Build history of the part. All positions in model axes, mm. A direction names the side the tool comes from. Round coordinates to 2 decimals unless told otherwise and drop trailing zeros. Write each loop counter-clockwise with the first axis right and the second up, starting at its lowest first coordinate (ties: lowest second). Pieces come first, ordered by that corner, then holes.
Item 1: 3-axis set-ups, long thin cutter, end or side, ignore diameter. For faces 4 (the flat face through (13, 17, -12)), 5 (the flat face through (0, 10, -10)), 6 (the conical face through (6.45, -4.125, -7.012)), 7 (the cylindrical face through (-11.77, 35.63, 9.85)), 8 (the flat face through (0, -6, -3)): which of +Z, -Z, +X, -X, +Y, -Y reach the whole face in a straight line?
Item 2: Drop flat-ended pins along their axis: pin 1 Ø14.5 at (x, y) = (-1, -17.5) entering from -Z; pin 2 Ø2 at (x, z) = (-4.5, -8) entering from -Y; pin 3 Ø1.8 at (x, z) = (9, -11) entering from +Y. Give the stop position or say it passes through.
Item 3: Wall check: probe 1 along X at (y, z) = (-13, 15); probe 2 along Y at (x, z) = (0, 15.3); probe 3 along Y at (x, z) = (-15, -4). Give the ranges that are in metal, low to high.
Item 4: Band-saw the part on A-A, the plane y = 3.5. Write the cut outline in (x, z), then the cut area to 3 significant figures.
Item 5: Band-saw the part on B-B, the plane y = 22. Write the cut outline in (x, z), then the cut area to 3 significant figures.
Item 6: Mould opens along X. For faces 1 (the conical face through (7.126, -4.125, 8.87)), 2 (the flat face through (0, 5, 10.5)), 3 (the flat face through (-20.5, 28, 0)) say: +X half, -X half, draft (parallel to the pull), parting line (faces both ways), or undercut.
Item 7: Band-saw the part on D-D, the plane x = 7.5. Count the separate pieces of the cut face and the enclosed holes in it, then the cut area to 3 significant figures.
```python
from build123d import *

# Parameters (mm, degrees)
F1_DEPTH  = 20.5
F2_R      = 1.5
F2_R_2    = 5
F3_DEPTH  = 6.001
F5_DEPTH  = 6
F6_R      = 1.5
F7_DEPTH  = 24.001
F8_SIZE   = 2
F9_R      = 1.5
F10_DEPTH = 38.001
F11_W     = 41
F11_H     = 38
F11_R     = 3
F11_R_2   = 1
F12_DEPTH = 19
F13_R     = 3
F14_DEPTH = 28
F16_DEPTH = 28
F17_R     = 4
F18_DEPTH = 9
F19_W     = 18
F19_H     = 18
F20_DEPTH = 18
F21_SIZE  = 17.99999
F22_SIZE  = 5
F24_DEPTH = 9
F25_R     = 4


# Not quite as in the source:
# - a fillet or chamfer is up to 0.001 mm smaller than in the source, because OpenCascade refuses the exact size


with BuildPart() as f1:
    # F0 (on Right) → F1 (new body, symmetric)
    with BuildSketch(Plane.YZ):
        Polygon((0, -10.5), (0, 10.5), (10, 10.5), (10, 9), (26, 9), (26, 19), (-20, 19), (-20, 13), (-6, 13), (-6, -19), (26, -19), (26, -9), (10, -9), (10, -10.5), align=None)
    extrude(amount=F1_DEPTH, both=True)

    # F2 (on face) → F3 (cut, through all)
    with BuildSketch(Plane(origin=(0, 0, 13), x_dir=(1, 0, 0), z_dir=(0, 0, -1))):
        with Locations((-8, 13)):
            Circle(F2_R)
        with Locations((8, 13)):
            Circle(F2_R)
        with Locations((0, 13)):
            Circle(F2_R_2)
    extrude(amount=-F3_DEPTH, mode=Mode.SUBTRACT)

    # F4 (on face) → F5 (join, through all)
    with BuildSketch(Plane.XY.offset(19)):
        with BuildLine():
            ThreePointArc((-8.4852813742, -20), (0, -24), (8.4852813742, -20))
            Line((8.4852813742, -20), (-8.4852813742, -20))
        make_face()
    extrude(amount=-F5_DEPTH)

    # F6 (on face) → F7 (cut, through all)
    with BuildSketch(Plane(origin=(0, 0, 0), x_dir=(-1, 0, 0), z_dir=(0, 1, 0))):
        with Locations((-8, 7.5)):
            Circle(F6_R)
        with Locations((8, 7.5)):
            Circle(F6_R)
        with Locations((8, -7.5)):
            Circle(F6_R)
        with Locations((-8, -7.5)):
            Circle(F6_R)
    extrude(amount=-F7_DEPTH, mode=Mode.SUBTRACT)

    # F8
    f8_edges = [f1.edges().sort_by_distance(p)[0] for p in [
        (-6.5, -6, 7.5),
        (9.5, -6, 7.5),
        (9.5, -6, -7.5),
        (-6.5, -6, -7.5),
    ]]
    chamfer(f8_edges, length=F8_SIZE)

    # F9 (on face) → F10 (cut, through all)
    with BuildSketch(Plane.XY.offset(19)):
        with Locations((-11, 22)):
            Circle(F9_R)
        with Locations((11, 22)):
            Circle(F9_R)
    extrude(amount=-F10_DEPTH, mode=Mode.SUBTRACT)

    # F11 (on face) → F12 (join)
    with BuildSketch(Plane(origin=(0, 26, 0), x_dir=(-1, 0, 0), z_dir=(0, 1, 0))):
        Rectangle(F11_W, F11_H)
        with Locations((-9, -11)):
            Circle(F11_R, mode=Mode.SUBTRACT)
        with Locations((-2.625, -3.5)):
            Circle(F11_R_2, mode=Mode.SUBTRACT)
        with Locations((2.625, 3.5)):
            Circle(F11_R_2, mode=Mode.SUBTRACT)
        with Locations((9, 11)):
            Circle(F11_R, mode=Mode.SUBTRACT)
    extrude(amount=F12_DEPTH)

    # F13 (on face) → F14 (cut)
    with BuildSketch(Plane(origin=(0, 45, 0), x_dir=(-1, 0, 0), z_dir=(0, 1, 0))):
        with Locations((9, 11)):
            Circle(F13_R)
        with Locations((-9, -11)):
            Circle(F13_R)
    extrude(amount=-F14_DEPTH, mode=Mode.SUBTRACT)

    # F15 (on face) → F16 (join, through all)
    with BuildSketch(Plane(origin=(0, 17, 0), x_dir=(-1, 0, 0), z_dir=(0, 1, 0))):
        with BuildLine():
            ThreePointArc((6.7639320225, 9), (9, 14), (11.2360679775, 9))
            Line((11.2360679775, 9), (20.5, 9))
            Line((20.5, 9), (20.5, 19))
            Line((20.5, 19), (0, 19))
            Line((0, 19), (0, 9))
            Line((0, 9), (6.7639320225, 9))
        make_face()
        with BuildLine():
            ThreePointArc((-6.7639320225, -9), (-9, -14), (-11.2360679775, -9))
            Line((-11.2360679775, -9), (-20.5, -9))
            Line((-20.5, -9), (-20.5, -19))
            Line((-20.5, -19), (0, -19))
            Line((0, -19), (0, -9))
            Line((0, -9), (-6.7639320225, -9))
        make_face()
    extrude(amount=F16_DEPTH)

    # F17 (on face) → F18 (cut, through all)
    with BuildSketch(Plane(origin=(0, 17, 0), x_dir=(-1, 0, 0), z_dir=(0, 1, 0))):
        with Locations((9, 11)):
            Circle(F17_R)
        with Locations((-9, -11)):
            Circle(F17_R)
    extrude(amount=F18_DEPTH, mode=Mode.SUBTRACT)

    # F19 (on face) → F20 (cut)
    with BuildSketch(Plane(origin=(0, 45, 0), x_dir=(-1, 0, 0), z_dir=(0, 1, 0))):
        with Locations((-11.5, 10)):
            Rectangle(F19_W, F19_H)
        with Locations((11.5, -10)):
            Rectangle(F19_W, F19_H)
    extrude(amount=-F20_DEPTH, mode=Mode.SUBTRACT)

    # F21 (size 18 in the source; OpenCascade refuses exactly that, so slightly less here)
    f21_edges = [f1.edges().sort_by_distance(p)[0] for p in [
        (2.5, 27, 10),
        (-2.5, 27, -10),
        (11.5, 27, 1),
        (2.5, 36, 1),
        (-2.5, 36, -1),
        (-11.5, 27, -1),
    ]]
    chamfer(f21_edges, length=F21_SIZE)

    # F22
    f22_edges = [f1.edges().sort_by_distance(p)[0] for p in [
        (20.5, -20, 16),
        (-20.5, -20, 16),
    ]]
    chamfer(f22_edges, length=F22_SIZE)

    # F23 (on face) → F24 (cut, through all)
    with BuildSketch(Plane.XZ.offset(-26)):
        with BuildLine():
            Line((20.5, -9), (12.4641016151, -9))
            ThreePointArc((12.4641016151, -9), (12.4641016151, -13), (9, -15))
            Line((9, -15), (20.5, -15))
            Line((20.5, -15), (20.5, -9))
        make_face()
        with BuildLine():
            Line((-20.5, 9), (-12.4641016151, 9))
            ThreePointArc((-12.4641016151, 9), (-12.4641016151, 13), (-9, 15))
            Line((-9, 15), (-20.5, 15))
            Line((-20.5, 15), (-20.5, 9))
        make_face()
    extrude(amount=F24_DEPTH, mode=Mode.SUBTRACT)

    # F25
    f25_edges = [f1.edges().sort_by_distance(p)[0] for p in [
        (-5.535898, 21.5, 9),
        (5.535898, 21.5, -9),
    ]]
    fillet(f25_edges, radius=F25_R)


solid = f1.part
```
Results:
1. face 4: +X
1. face 5: +X, -X
1. face 6: -Y
1. face 7: +Y
1. face 8: -Z, +X, -X, -Y
2. pin 1: stops at z = 13
2. pin 2: stops at y = -6
2. pin 3: stops at y = 17
3. probe 1: x = -20.5 to -9.5, -6.5 to -5, 5 to 6.5, 9.5 to 20.5
3. probe 2: y = -24 to -18, -8 to 45
3. probe 3: y = -6 to 0, 26 to 45
4. outline: (-20.5, -19) - (20.5, -19) - (20.5, -10.5) - (-20.5, -10.5) - close; (-20.5, 10.5) - (20.5, 10.5) - (20.5, 19) - (-20.5, 19) - close
4. area: 697 mm2
5. outline: (-20.5, -19) - (-12.5, -19) - (-12.5, -9) - (-20.5, -9) - close; (-20.5, 15) - (-9, 15) arc R4 cw to (-5.13, 12) arc R4 ccw to (-1.25, 9) - (9.5, 9) - (9.5, 19) - (-20.5, 19) - close; (-9.5, -19) - (20.5, -19) - (20.5, -15) - (9, -15) arc R4 cw to (5.13, -12) arc R4 ccw to (1.25, -9) - (-9.5, -9) - close; (12.5, 9) - (20.5, 9) - (20.5, 19) - (12.5, 19) - close
5. area: 576 mm2
6. face 1: undercut
6. face 2: draft
6. face 3: -X half
7. separate pieces: 4
7. enclosed holes: 0
7. area: 1,310 mm2
